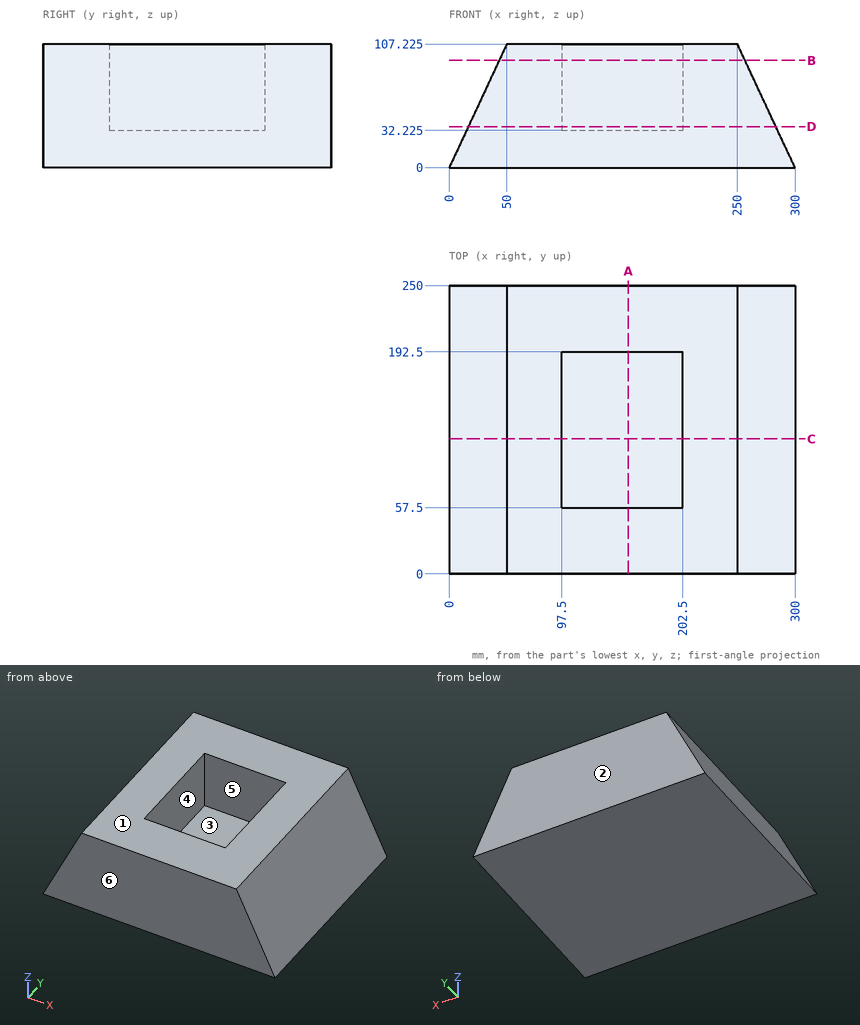
Input: dimensioned drawing with shaded views. Units: mm. Origin: part minimum x, y, z. A direction names the side the tool comes from. Round coordinates to 2 decimals unless told otherwise and drop trailing zeros. Order: outer loops, then holes, each group sorted by start corner. A loop starts at its lowest first (then second) coordinate and runs counter-clockwise, first axis right, second up.
Q1. Section B-B, the plane z = 93. Output: boundary loops of the cut face in (x, y).
Result sheet:
outline: (43.37, 0) - (256.63, 0) - (256.63, 250) - (43.37, 250) - close; hole (97.5, 57.5) - (202.5, 57.5) - (202.5, 192.5) - (97.5, 192.5) - close
Q2. Access query for the marked faces 5 and 6. Directions: +Z, -Z, +X, -X, +Y, -Y. A direction counts if a zero-diameter tool reaches every point of the face in a straight line with its end or side. Return the directions, or none.
Result sheet:
face 5: +Z
face 6: +Z, -Z, +X, -X, -Y
Q3. Mould query, pull axis Y, two halves, no side actions, for the marked faces 1, 2, 3 and 4. Classes: released by +Y, released by -Y, zero draft, split by the parting line, or undercut.
Result sheet:
face 1: zero draft
face 2: released by +Y
face 3: undercut
face 4: undercut
Q4. Section C-C, the plane y = 117. Output: boundary loops of the cut face in (x, z) (1 decimal), and give its area (3 significant figures).
Result sheet:
outline: (0, 0) - (300, 0) - (250, 107.2) - (202.5, 107.2) - (202.5, 32.2) - (97.5, 32.2) - (97.5, 107.2) - (50, 107.2) - close
area: 18,900 mm2
Q5. Section D-D, the plane z = 35.5. Output: boundary loops of the cut face in (x, y), and give its area (3 significant figures).
Result sheet:
outline: (16.55, 0) - (283.45, 0) - (283.45, 250) - (16.55, 250) - close; hole (97.5, 57.5) - (202.5, 57.5) - (202.5, 192.5) - (97.5, 192.5) - close
area: 52,500 mm2
Q6. Material intervals for probe 1 along Y at (x, z) = (160, 85); probe 2 along Z at (x, y) = (104.5, 178.5) (1 decimal); probe 3 along X at (y, z) = (152, 44.5), sorted ascending.
Result sheet:
probe 1: y = 0 to 57.5, 192.5 to 250
probe 2: z = 0 to 32.2
probe 3: x = 20.75 to 97.5, 202.5 to 279.25
Q7. Pin query (flat end, axial travel): pin 1 (22.5 mm diameter, centred on y = 134.5, z = 71.5, fed in from -X) (1 decimal); pin 2 (12 mm diameter, centred on y = 55.5, z = 58, fed in from +X); pin 3 (12 mm diameter, centred on y = 29, z = 69.5, fed in from +X); pin 4 (2 mm diameter, centred on x = 260, z = 34, fed in from -Y). Return the tip coordinate at first contact, or that it passes through.
Result sheet:
pin 1: stops at x = 28.1
pin 2: stops at x = 275.75
pin 3: stops at x = 270.39
pin 4: stops at y = 0
Q8. Section A-A, the plane x = 155.5. Output: boundary loops of the cut face in (y, z) (1 decimal).
Result sheet:
outline: (0, 0) - (250, 0) - (250, 107.2) - (192.5, 107.2) - (192.5, 32.2) - (57.5, 32.2) - (57.5, 107.2) - (0, 107.2) - close
